from build123d import *

# Parameters (mm, degrees)
SKETCH006_W             = 35.6
SKETCH006_H             = 11.6
PAD006_DEPTH            = 55.8
SKETCH007_W             = 34
SKETCH007_H             = 10
POCKET_DEPTH            = 55
SKETCH008_W             = 3
SKETCH008_H             = 3
POCKET001_DEPTH         = 3
BODY001_PLACEMENT_ANGLE = 90


with BuildPart() as part:
    # Sketch006 → Pad006 (new body)
    with BuildSketch(Plane.XZ):
        Rectangle(SKETCH006_W, SKETCH006_H)
    extrude(amount=PAD006_DEPTH)

    # Sketch007 → Pocket (cut)
    with BuildSketch(Plane.XZ):
        Rectangle(SKETCH007_W, SKETCH007_H)
    extrude(amount=POCKET_DEPTH, mode=Mode.SUBTRACT)

    # Sketch008 → Pocket001 (cut)
    with BuildSketch(Plane.XZ):
        with Locations((-16.3, 4.3)):
            Rectangle(SKETCH008_W, SKETCH008_H)
        with Locations((16.3, -4.3)):
            Rectangle(SKETCH008_W, SKETCH008_H)
        with Locations((-16.3, 0)):
            Rectangle(SKETCH008_W, SKETCH008_H)
        with Locations((16.3, 0)):
            Rectangle(SKETCH008_W, SKETCH008_H)
    extrude(amount=POCKET001_DEPTH, mode=Mode.SUBTRACT)


with BuildPart() as part_1:
    # Body001 placement: moved
    add(part.part.moved(Location((27, -12.5, 0.5))).rotate(Axis((27, -12.5, 0.5), (0, 0, -1)), BODY001_PLACEMENT_ANGLE))


solid = part_1.part
Part model, mm, in its own coordinate system. A direction names the side the tool comes from. Coordinates: 2 decimals unless noted, no trailing zeros. Order: outer loops, then holes, each group sorted by start corner. A loop starts at its lowest first (then second) coordinate and runs counter-clockwise, first axis right, second up. Notation, with made-up numbers: M -34.75,14 L -22.75,14 A26 cw -22.75,51 Z; hole C 11.5,30 d9. An arc over 180 degrees is marked long. One line per question, with ' | ' between items.
Q1. Pin check, flat tips, straight feed: P1, Ø1.5, axis at y = -28.5, z = -4, coming from the +X side; P2, Ø0.6, axis at x = 26, y = -30, coming from the -Z side; P3, Ø0.6, axis at x = 25, z = 6, coming from the +Y side. Stop position of each tip, or through.
A:
P1: stops at x = 24 | P2: stops at z = -2.3 | P3: stops at y = 2.3
Q2. Slice it at B-B (x = -3). Give the cut face in (y, z).
A:
outline: M -30.3,-5.3 L 5.3,-5.3 L 5.3,6.3 L -30.3,6.3 Z; hole M -29.5,-4.5 L 4.5,-4.5 L 4.5,5.5 L -29.5,5.5 Z
Q3. Drill centre lines: line 1 (Y direction, x = -22.5, z = -0.25); line 2 (Z direction, x = 9, y = -21); line 3 (X direction, y = -22.5, z = 4.75). Where is each one in solid material? Low to high.
A:
line 1: y = -30.3 to -29.5, 4.5 to 5.3 | line 2: z = -5.3 to -4.5, 5.5 to 6.3 | line 3: x = -28.8 to -28
Q4. 3-axis set-ups, long thin cutter, end or side, ignore diameter. For faces 5 (the face through (24, -30, -4)), 6 (the face through (0, 4.5, 0)), 7 (the face through (24, 4, 6)): which of +Z, -Z, +X, -X, +Y, -Y reach the whole face in a straight line?
A:
face 5: -Z, +X, -Y | face 6: +X | face 7: +Z, +X, +Y
Q5. Slice it at C-C (y = -22). Give the cut face in (x, z).
A:
outline: M -28.8,-5.3 L 27,-5.3 L 27,-4.5 L -28,-4.5 L -28,5.5 L 27,5.5 L 27,6.3 L -28.8,6.3 Z
Q6. Two-plate mould, pull along Z, no slides. Class faces 1 (the face through (0, -29.5, 0)), 2 (the face through (-1, -12, 6.3)), 3 (the face through (27, -16, 6)), 4 (the face through (-1, -12, -5.3)): +Z half, -Z half, draft (parallel to the pull), parting line (faces both ways), or undercut.
A:
face 1: undercut | face 2: +Z half | face 3: draft | face 4: -Z half
Q7. Slice it at A-A (z = 0.25). Give the cut face in (x, y), and give its area (3 significant figures).
A:
outline: M -28.8,-30.3 L 24,-30.3 L 24,-29.5 L -28,-29.5 L -28,4.5 L 24,4.5 L 24,5.3 L -28.8,5.3 Z | area: 112 mm^2
